Design review of the part built by this model. Coordinates are the model's own, in mm. Coordinates: 2 decimals unless noted, no trailing zeros. Order: outer loops, then holes, each group sorted by start corner. A loop starts at its lowest first (then second) coordinate and runs counter-clockwise, first axis right, second up. Notation, with made-up numbers: M -4.5,25 L 25.5,25 A26 cw 25.5,52 Z; hole C -23.75,75.5 d8. An arc over 180 degrees is marked long. Answer as a JSON object with one key per item and string values.
from build123d import *

# Parameters (mm, degrees)
BOSS_EXTRUDE1_DEPTH = 3.81
SKETCH2_R           = 1.65
CUT_EXTRUDE1_DEPTH  = 8.89
SKETCH3_R           = 1.75
CUT_EXTRUDE2_DEPTH  = 154.633260071


with BuildPart() as part:
    # Sketch1 → Boss-Extrude1 (new body)
    with BuildSketch(Plane.XY):
        Polygon((-107.95, -76.2), (-133.35, -50.8), (-133.35, 50.8), (-107.95, 76.2), (19.05, 76.2), (19.05, -76.2), align=None)
    extrude(amount=BOSS_EXTRUDE1_DEPTH)

    # Sketch2 → Cut-Extrude1 (cut)
    with BuildSketch(Plane.XY.offset(3.81)):
        with Locations((1.75833287, 57.577017073)):
            Circle(SKETCH2_R)
        with Locations((-14.239074115, 57.577017073)):
            Circle(SKETCH2_R)
        with Locations((-92.542171462, 57.577017073)):
            Circle(SKETCH2_R)
        with Locations((-108.82023471, 57.577017073)):
            Circle(SKETCH2_R)
        with Locations((-108.82023471, -57.577017073)):
            Circle(SKETCH2_R)
        with Locations((-92.542171462, -57.577017073)):
            Circle(SKETCH2_R)
        with Locations((-14.239074115, -57.577017073)):
            Circle(SKETCH2_R)
        with Locations((1.75833287, -57.577017073)):
            Circle(SKETCH2_R)
    extrude(amount=-CUT_EXTRUDE1_DEPTH, mode=Mode.SUBTRACT)

    # Sketch3 → Cut-Extrude2 (cut, through all)
    with BuildSketch(Plane.XY.offset(3.81)):
        with Locations((-80.308350336, 29.360206552)):
            Circle(SKETCH3_R)
        with Locations((-17.285686927, 31.245112915)):
            Circle(SKETCH3_R)
        with Locations((-17.285686927, -30.956551268)):
            Circle(SKETCH3_R)
        with Locations((-80.308350336, -29.071644905)):
            Circle(SKETCH3_R)
    extrude(amount=-CUT_EXTRUDE2_DEPTH, mode=Mode.SUBTRACT)


solid = part.part
1) Mouldability with a two-part tool opening along X and no side actions: class faces 1 (the cylindrical face through (-107.246, 58.073, 1.932)), 2 (the cylindrical face through (-107.296, -58.209, 1.932)), 3 (the flat face through (-120.83, 63.32, 1.88)), 4 (the flat face through (19.05, 1, 2)) as released by +X, released by -X, zero draft, split by the parting line, or undercut.
Taken from the geometry:
{"face 1": "undercut", "face 2": "undercut", "face 3": "released by -X", "face 4": "released by +X"}
2) Add section A-A (z = 0.6). Count the separate pieces of the cut face and the enclosed holes in it, and give its area (3 significant figures).
Taken from the geometry:
{"separate pieces": "1", "enclosed holes": "12", "area": "22,500 mm2"}
3) To check wall thickness, follow L1, parallel to Y at x = 1.5, z = 1.1; L2, parallel to X at y = 28.5, z = 3.2; L3, parallel to X at y = -30, z = 0.5. State the ranges of each line that lie inside material, in increasing order.
Taken from the geometry:
{"L1": "y = -76.2 to -59.21, -55.95 to 55.95, 59.21 to 76.2", "L2": "x = -133.35 to -81.83, -78.78 to 19.05", "L3": "x = -133.35 to -81.79, -78.82 to -18.75, -15.82 to 19.05"}
4) Add section B-B (y = 63). State the section outline as (x, z) points, and give its area (3 significant figures).
Taken from the geometry:
{"outline": "M -121.15,0 L 19.05,0 L 19.05,3.81 L -121.15,3.81 Z", "area": "534 mm2"}
